Design review of the part shown in the three views and the two pictorial views. Dimensions are in mm from the part's minimum x, y and z. Coordinates: 2 decimals unless noted, no trailing zeros. Loops run counter-clockwise (first coordinate to the right, second up) from the corner with the lowest first, then second, coordinate; pieces in that order, holes last. Notation, with made-up numbers: M 67,-12.75 L 115,-12.75 A38 ccw 115,26.25 Z; hole C -33.75,47.5 d7. An arc over 180 degrees is marked long. Write item = value, one per line. Start each with the question number.
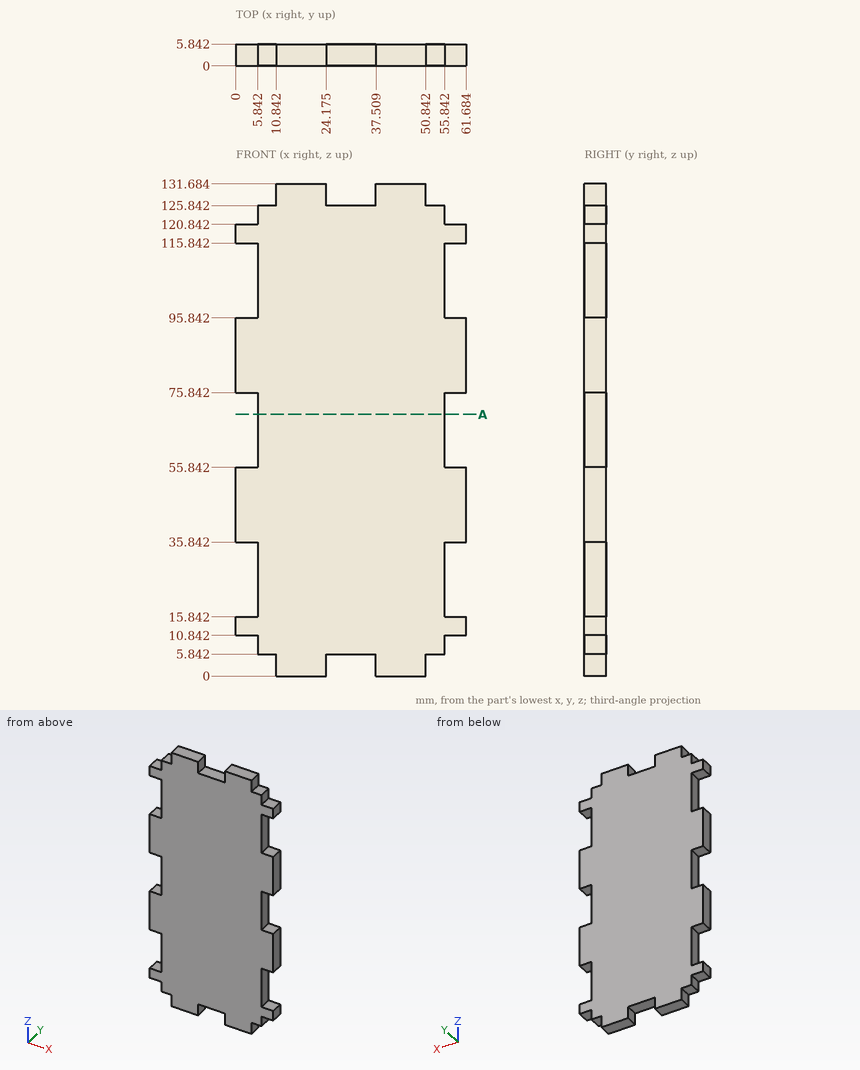
(1) To check wall thickness, follow L1, parallel to Z at x = 5, y = 1; L2, parallel to Z at x = 32.5, y = 3.7; L3, parallel to X at y = 0.5, z = 21. State the ranges of each line that lie inside material, in increasing order.
(2) Insertion check: pin 1 (3 mm diameter, centred on y = 3, z = 127.5, fed in from -X); pin 2 (3 mm diameter, centred on y = 3, z = 111, fed in from +X); pin 3 (3 mm diameter, centred on x = 58.5, y = 2.5, fed in from -Z); pin 4 (1 mm diameter, centred on x = 45.5, y = 3, fed in from -Z). Each pin has a flat end and moves straight along its axis. Give the tip position at first contact, or say it passes through.
(3) Take a section at A-A (z = 70). State the section outline as (x, y) points, plus the area to 3 significant figures.
Results list:
q1.L1 = 10.84 to 15.84, 35.84 to 55.84, 75.84 to 95.84, 115.84 to 120.84
q1.L2 = 5.84 to 125.84
q1.L3 = 5.84 to 55.84
q2.pin_1 = 10.84
q2.pin_2 = 55.84
q2.pin_3 = 10.84
q2.pin_4 = 0
q3.outline = M 5.84,0 L 55.84,0 L 55.84,5.84 L 5.84,5.84 Z
q3.area = 292 mm^2
